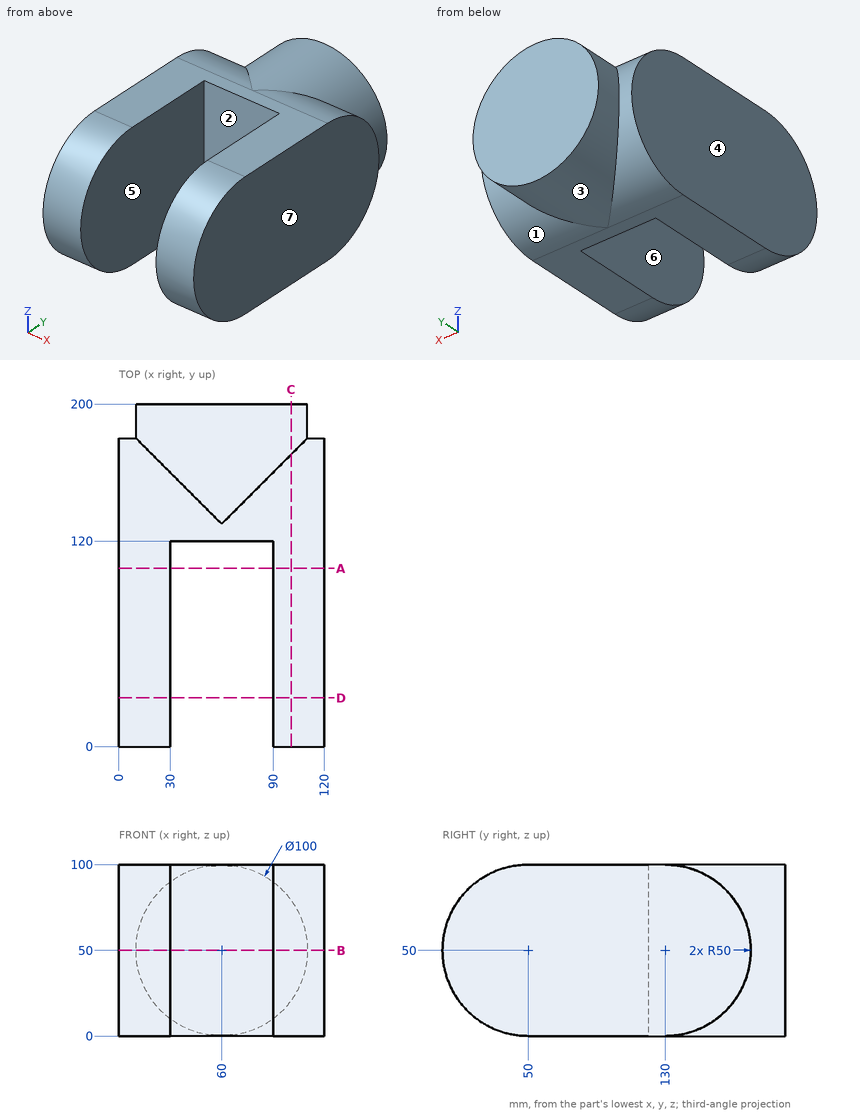
Geometry: see drawing. Coordinates: mm, zero at the bounding-box minimum. A direction names the side the tool comes from. Give positions to 0.01 mm unless a question says otherwise; leave off trailing zeros. Loops run counter-clockwise (first coordinate to the right, second up) from the corner with the lowest first, then second, coordinate; pieces in that order, holes last. Notation, with made-up numbers: (80, 72.5) -> (98, 72.5) arc R19 cw to (98, 98.5) -> close; hole circle Ø8 at (-1.75, 41). An arc over 180 degrees is marked (long way). Answer as a JSON object with one key per item and string values. Group by question number.
Item 1: Cut plane B-B, the plane z = 50. Return the cut outline in (x, y), and give its area (3 significant figures).
Item 2: Pull-direction query (X, two-part tool) for the marked faces 4, 5, 6 and 7; classes: released by +X, released by -X, zero draft, split by the parting line, or undercut.
Item 3: Cut plane C-C, the plane x = 100.5. Return the cut outline in (y, z), and give its area (3 significant figures).
Item 4: Cut plane D-D, the plane y = 28.5. Return the cut outline in (x, z).
Item 5: Pin query (flat end, axial travel): P1, Ø4, axis at x = 77.5, y = 157.5, coming from the +Z side; P2, Ø1.5, axis at x = 100.5, z = 86.5, coming from the +Y side; P3, Ø5, axis at x = 25, y = 142.5, coming from the -Z side. Return the tip coordinate at first contact, or that it passes through.
Item 6: Line query: probe 1 along X at (y, z) = (51, 30); probe 2 along Y at (x, z) = (51, 84); probe 3 along Y at (x, z) = (12.5, 72.5). Output: solid intervals per line, ascending.
Item 7: Cut plane A-A, the plane y = 104. Return the cut outline in (x, z).
Item 8: Reachability of the marked faces 1, 2 and 3 from +Z, -Z, +X, -X, +Y, -Y: full face, straight path, thin tool, end or side. Return the list, or none.
Checks:
{
 "1": {"outline": "(0, 0) -> (30, 0) -> (30, 120) -> (90, 120) -> (90, 0) -> (120, 0) -> (120, 180) -> (110, 180) -> (110, 200) -> (10, 200) -> (10, 180) -> (0, 180) -> close", "area": "16,400 mm²"},
 "2": {"face 4": "released by -X", "face 5": "undercut", "face 6": "undercut", "face 7": "released by +X"},
 "3": {"outline": "(50, 0) -> (130, 0) arc R50 ccw to (170.5, 20.68) -> (200, 20.68) -> (200, 79.32) -> (170.5, 79.32) arc R50 ccw to (130, 100) -> (50, 100) arc R50 ccw to start", "area": "17,200 mm²"},
 "4": {"outline": "(0, 4.86) -> (30, 4.86) -> (30, 95.14) -> (0, 95.14) -> close; (90, 4.86) -> (120, 4.86) -> (120, 95.14) -> (90, 95.14) -> close"},
 "5": {"P1": "stops at z = 97.54", "P2": "stops at y = 164.96", "P3": "stops at z = 1.01"},
 "6": {"probe 1": "x = 0 to 30, 90 to 120", "probe 2": "y = 120 to 200", "probe 3": "y = 5.35 to 174.65"},
 "7": {"outline": "(0, 0) -> (30, 0) -> (30, 100) -> (0, 100) -> close; (90, 0) -> (120, 0) -> (120, 100) -> (90, 100) -> close"},
 "8": {"face 1": "+X, +Y", "face 2": "+Z, -Z, -Y", "face 3": "+Y"}
}
